Here's how the part is built. I have some questions about the finished solid (model axes, mm). Face numbers are marked on the shaded views. A direction names the side the tool comes from. Coordinates: 2 decimals unless noted, no trailing zeros. Loops run counter-clockwise (first coordinate to the right, second up) from the corner with the lowest first, then second, coordinate; pieces in that order, holes last. Notation, with made-up numbers: (24.25, 63.25) -> (45.25, 63.25) arc R23 cw to (45.25, 95.25) -> close; hole circle Ø2 at (60.25, 28). An arc over 180 degrees is marked (long way). Answer as a JSON object with one key per item and string values. Group by question number.
Q1. I need wall thicknesses on line 1 (X direction, y = 1.75, z = -2) (3 decimals); line 2 (Z direction, x = 2.5, y = 12); line 3 (Y direction, x = 4.5, z = -6.5). Which ranges of each line are inside material? Lowest first, please.
Q2. Thinking about a two-plate mould opening in X: for the marked faces 1, 2 and 3, which applies, released by +X, released by -X, zero draft, split by the parting line, or undercut?
Q3. On a 3-axis mill with a long thin cutter (end or side, diameter ignored), from which of +Z, -Z, +X, -X, +Y, -Y can I reach the whole of each face in a straight line? I mean the marked faces 4 and 5. Say none if no direction works.
Q4. I want a section at C-C on x = 4.75. Count the separate pieces of the cut face and the enclosed holes in it, then the cut area to 3 significant figures.
Q5. I want a section at D-D on y = 3.75. Write out the boundary of the cut face in (x, z).
Q6. I want a section at B-B on z = -15. Write out the boundary of the cut face in (x, y) (3 decimals).
Q7. I want a section at A-A on y = 14.5. Write out the boundary of the cut face in (x, z) (3 decimals).
Q8. I'm going to push flat-ended pins straight in: pin 1 (2 mm diameter, centred on x = 5, y = 12.5, fed in from +Z); pin 2 (3.5 mm diameter, centred on x = 1.875, z = -15, fed in from +Y). Where does each tip first touch, or does it pass through?
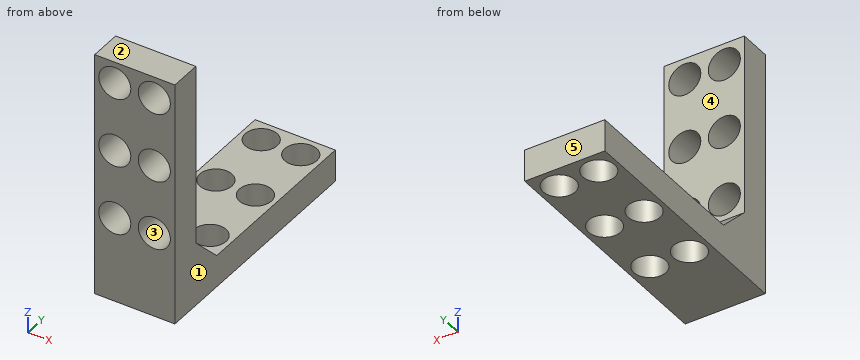
```python
from build123d import *

# Parameters (mm, degrees)
BOSS_EXTRUDE1_DEPTH  = 7.5
CHAMFER1_SIZE        = 3
SKETCH3_R            = 1.5
CUT_EXTRUDE1_DEPTH   = 10
SKETCH4_R            = 1.5
CUT_EXTRUDE2_DEPTH   = 10
LPATTERN1_COUNT      = 2
LPATTERN1_PITCH      = 3.7
LPATTERN1_COUNT_DIR2 = 5
LPATTERN1_PITCH_DIR2 = 3.25
LPATTERN2_COUNT      = 2
LPATTERN2_PITCH      = 3.7
LPATTERN2_COUNT_DIR2 = 5
LPATTERN2_PITCH_DIR2 = 3.25


with BuildPart() as part:
    # Sketch1 → Boss-Extrude1 (new body)
    with BuildSketch(Plane(origin=(0, 0, 0), x_dir=(0, 0, -1), z_dir=(1, 0, 0))):
        Polygon((0, 0), (0, 3), (20, 3), (20, 23), (23, 23), (23, 0), align=None)
    extrude(amount=BOSS_EXTRUDE1_DEPTH)

    # Chamfer1
    chamfer1_edges = [part.edges().sort_by_distance(p)[0] for p in [
        (3.75, 3, -20),
    ]]
    chamfer(chamfer1_edges, length=CHAMFER1_SIZE)

    # Sketch3 → Cut-Extrude1 (cut)
    with BuildSketch(Plane.XY.offset(-20)):
        with Locations((1.875, 21)):
            Circle(SKETCH3_R)
    cut_extrude1 = extrude(amount=-CUT_EXTRUDE1_DEPTH, mode=Mode.SUBTRACT)

    # Sketch4 → Cut-Extrude2 (cut)
    with BuildSketch(Plane(origin=(0, 3, 0), x_dir=(1, 0, 0), z_dir=(0, 1, 0))):
        with Locations(Location((1.875, 2, 0), (0, 0, 270))):
            Circle(SKETCH4_R)
    cut_extrude2 = extrude(amount=-CUT_EXTRUDE2_DEPTH, mode=Mode.SUBTRACT)

    # LPattern1: Cut-Extrude1 2 × 5, 4 skipped
    with Locations(*[(i * LPATTERN1_PITCH, -j * LPATTERN1_PITCH_DIR2, 0) for i in range(LPATTERN1_COUNT) for j in range(LPATTERN1_COUNT_DIR2) if (i, j) not in ((0, 0), (0, 1), (0, 3), (1, 1), (1, 3))]):
        add(cut_extrude1, mode=Mode.SUBTRACT)

    # LPattern2: Cut-Extrude2 2 × 5, 4 skipped
    with Locations(*[(i * LPATTERN2_PITCH, 0, -j * LPATTERN2_PITCH_DIR2) for i in range(LPATTERN2_COUNT) for j in range(LPATTERN2_COUNT_DIR2) if (i, j) not in ((0, 0), (0, 1), (0, 3), (1, 1), (1, 3))]):
        add(cut_extrude2, mode=Mode.SUBTRACT)


solid = part.part
```
Result set:
{
 "1": {"line 1": "x = 0 to 0.375, 3.375 to 4.075, 7.075 to 7.5", "line 2": "z = -23 to -20", "line 3": "y = 0 to 3"},
 "2": {"face 1": "released by +X", "face 2": "zero draft", "face 3": "undercut"},
 "3": {"face 4": "+Z, +X, -X, +Y", "face 5": "+Z, -Z, +X, -X, +Y"},
 "4": {"separate pieces": "7", "enclosed holes": "0", "area": "88.4 mm²"},
 "5": {"outline": "(0, -23) -> (7.5, -23) -> (7.5, -17.75) -> (0, -17.75) -> close"},
 "6": {"outline": "(0, 0) -> (0.375, 0) -> (0.375, 3) -> (0, 3) -> close; (3.375, 0) -> (4.075, 0) -> (4.075, 3) -> (3.375, 3) -> close; (7.075, 0) -> (7.5, 0) -> (7.5, 3) -> (7.075, 3) -> close"},
 "7": {"outline": "(0, -23) -> (0.375, -23) -> (0.375, -20) -> (0, -20) -> close; (3.375, -23) -> (4.075, -23) -> (4.075, -20) -> (3.375, -20) -> close; (7.075, -23) -> (7.5, -23) -> (7.5, -20) -> (7.075, -20) -> close"},
 "8": {"pin 1": "stops at z = -20", "pin 2": "stops at y = 3"}
}
